Design review of the part shown in the three views and the two pictorial views. Dimensions are in mm from the part's minimum x, y and z. Give positions to 0.01 mm unless a question says otherwise; leave off trailing zeros. Loops run counter-clockwise (first coordinate to the right, second up) from the corner with the lowest first, then second, coordinate; pieces in that order, holes last. Notation, with made-up numbers: (68.25, 79.5) - (105.25, 79.5) arc R20 cw to (105.25, 94.5) - close; hole circle Ø1 at (-12, 27.5). An arc over 180 degrees is marked (long way). Put each result on its own line as item: value. Start each with the question number.
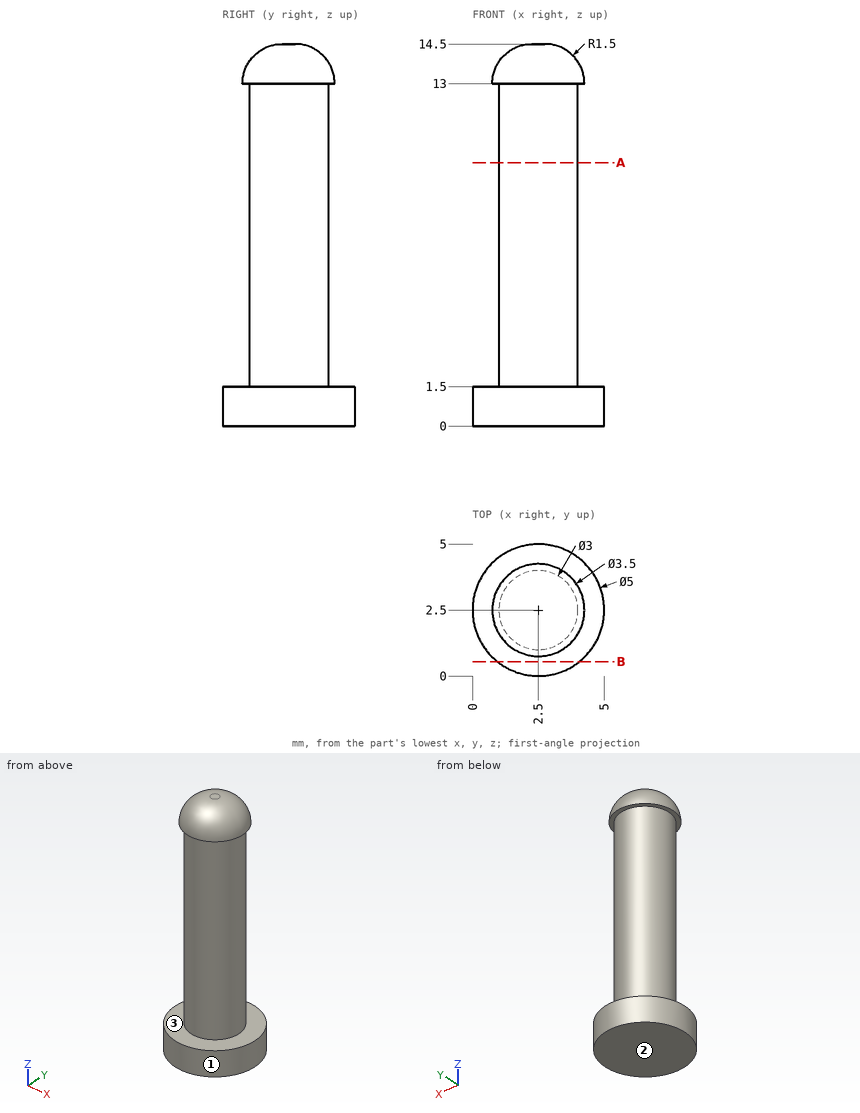
1) Insertion check: P1, Ø1.5, axis at y = 1, z = 6.5, coming from the +X side; P2, Ø1, axis at y = 1, z = 13, coming from the +X side. Each pin has a flat end and moves straight along its axis. Give the tip position at first contact, or say it passes through.
2) Take a section at A-A on z = 10. State the section outline as (x, y) points.
3) Mouldability with a two-part tool opening along Z and no side actions: class the marked faces 1, 2 and 3 as released by +Z, released by -Z, zero draft, split by the parting line, or undercut.
4) Wall thickness on probe 1 along Z at (x, y) = (1.5, 0.25); probe 2 along Z at (x, y) = (2.1, 4.05); probe 3 along Y at (x, z) = (2.55, 4.5): over which ranges is each line inside the solid? List them lowest first.
5) Take a section at B-B on y = 0.55. State the section outline as (x, z) points, and give its area (3 significant figures).
Answers follow:
1. P1: x = 3.8
1. P2: x = 3.94
2. outline: circle Ø3 at (2.5, 2.5)
3. face 1: zero draft
3. face 2: released by -Z
3. face 3: undercut
4. probe 1: 0 to 1.5
4. probe 2: 0 to 1.5, 13 to 13.65
4. probe 3: 1 to 4
5. outline: (0.94, 0) - (4.06, 0) - (4.06, 1.5) - (0.94, 1.5) - close
5. area: 4.69 mm2
